Part model, mm, in its own coordinate system. Give positions to 0.01 mm unless a question says otherwise; leave off trailing zeros. Order: outer loops, then holes, each group sorted by start corner. A loop starts at its lowest first (then second) coordinate and runs counter-clockwise, first axis right, second up. Notation, with made-up numbers: (49, 59.5) - (74, 59.5) arc R10 ccw to (74, 71.5) - close; hole circle Ø11 at (-3.5, -3). An arc over 180 degrees is marked (long way). Use one line per item in the form item = value. Start each with the question number.
1. Pin check, flat tips, straight feed: P1, Ø0.9, axis at x = -322, y = 2, coming from the -Z side; P2, Ø0.9, axis at y = 1, z = 170.5, coming from the -X side; P3, Ø1.5, axis at x = -310.5, y = 2, coming from the +Z side. Stop position of each tip, or through.
2. Band-saw the part on A-A, the plane y = 0.9. List the corners of the cut face in (x, z), plus the area to 3 significant figures.
3. Drill centre lines: line 1 (Z direction, x = -336, y = 1.25); line 2 (X direction, y = 2.15, z = 171). Where is each one in solid material? Low to high.
4. Band-saw the part on B-B, the plane x = -179. List the corners of the cut face in (y, z), plus the area to 3 significant figures.
Autodesk Inventor part; units mm, degrees
ref_plane "YZ Plane" through (0, 0, 0) normal (1, 0, 0) x (0, 1, 0)
ref_plane "XZ Plane" through (0, 0, 0) normal (0, 1, 0) x (-1, 0, 0)
ref_plane "XY Plane" through (0, 0, 0) normal (0, 0, 1) x (1, 0, 0)
sketch "Sketch1" plane through (0, 0, 0) normal (0, 1, 0) x (-1, 0, 0)
  line L0 (374.9202, 193.7426) -> (-387.0798, 193.7426)
  line L1 (-387.0798, 193.7426) -> (-387.0798, -263.4574)
  line L2 (-387.0798, -263.4574) -> (374.9202, -263.4574)
  line L3 (374.9202, -263.4574) -> (374.9202, 193.7426)
  point P0 (0, 0)
  dimension "d0" = 457.2
  dimension "d1" = 762
extrude "Extrusion1" add sketch "Sketch1" along normal blind 2.9972
sketch "Sketch3" plane through (0, 2.9972, 0) normal (0, 1, 0) x (1, 0, 0)
  line L0 (-374.9202, 212.6574) -> (-171.7202, 212.6574)
  line L1 (-171.7202, 212.6574) -> (-171.7202, 263.4574)
  line L2 (-171.7202, 263.4574) -> (-374.9202, 263.4574)
  line L3 (-374.9202, 263.4574) -> (-374.9202, 212.6574)
  line L4 (-374.9202, 263.4574) -> (-374.9202, -193.7426)
  line L5 (-374.9202, -193.7426) -> (-171.7202, -193.7426)
  line L6 (-171.7202, -193.7426) -> (-171.7202, -142.9426)
  line L7 (-171.7202, -142.9426) -> (-374.9202, -142.9426)
  line L8 (-374.9202, -142.9426) -> (-374.9202, -193.7426)
  line L9 (387.0798, 263.4574) -> (-374.9202, 263.4574)
  line L10 (387.0798, -193.7426) -> (387.0798, 263.4574)
  point P0 (0, 0)
  point P1 (-374.9202, -142.9426)
  dimension "d9" = 50.8
  dimension "d12" = 203.2
extrude "Extrusion3" cut sketch "Sketch3" against normal through all
properties part number "2021 Underbelly" material "Polycarbonate, Clear"
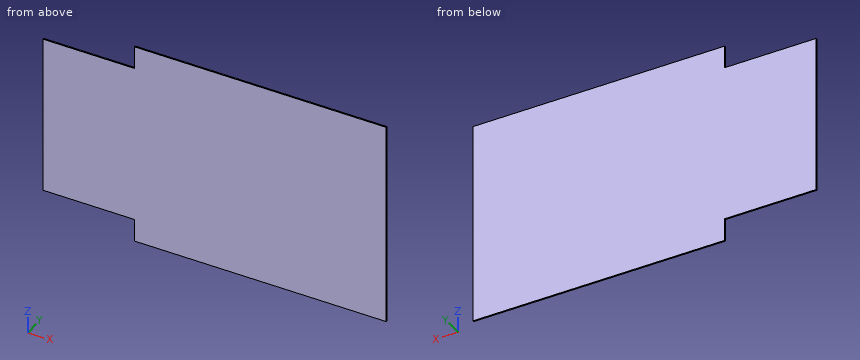
From the geometry:
q1.P1 = -212.66
q1.P2 = -171.72
q1.P3 = 142.94
q2.outline = (-374.92, -212.66) - (-171.72, -212.66) - (-171.72, -263.46) - (387.08, -263.46) - (387.08, 193.74) - (-171.72, 193.74) - (-171.72, 142.94) - (-374.92, 142.94) - close
q2.area = 328,000 mm²
q3.line_1 = -212.66 to 142.94
q3.line_2 = -171.72 to 387.08
q4.outline = (0, -212.66) - (3, -212.66) - (3, 142.94) - (0, 142.94) - close
q4.area = 1,070 mm²
